Here's how the part is built. I have some questions about the finished solid (model axes, mm). Give positions to 0.01 mm unless a question says otherwise; leave off trailing zeros. Order: outer loops, then holes, each group sorted by start corner. A loop starts at its lowest first (then second) coordinate and runs counter-clockwise, first axis right, second up. Notation, with made-up numbers: M 4.5,56.25 L 40.5,56.25 A22 ccw 40.5,89.25 Z; hole C 61,56 d2. An arc over 180 degrees is marked long. One line per item, written item: value. Start each with the question number.
from build123d import *

# Parameters (mm, degrees)
SKETCH1_R           = 1.5
SKETCH1_R_2         = 3.75
BOSS_EXTRUDE1_DEPTH = 3


with BuildPart() as part:
    # Sketch1 → Boss-Extrude1 (new body)
    # profile 1 of 3: a face of its own
    with BuildSketch(Plane.XY):
        with BuildLine():
            Line((40, 3.75), (0, 3.75))
            ThreePointArc((0, 3.75), (2.651650429, 2.651650429), (3.75, 0))
            ThreePointArc((3.75, 0), (2.651650429, -2.651650429), (0, -3.75))
            Line((0, -3.75), (40, -3.75))
            ThreePointArc((40, -3.75), (36.25, 0), (40, 3.75))
        make_face()
        with Locations((32, 0)):
            Circle(SKETCH1_R, mode=Mode.SUBTRACT)
    # profile 2 of 3: a face of its own
    with BuildSketch(Plane.XY):
        Circle(SKETCH1_R_2)
        Circle(SKETCH1_R, mode=Mode.SUBTRACT)
    # profile 3 of 3: a face of its own
    with BuildSketch(Plane.XY):
        with Locations((40, 0)):
            Circle(SKETCH1_R_2)
        with Locations((40, 0)):
            Circle(SKETCH1_R, mode=Mode.SUBTRACT)
    extrude(amount=BOSS_EXTRUDE1_DEPTH)


solid = part.part
Item 1: I want a section at C-C on x = 32. Write out the boundary of the cut face in (y, z).
Item 2: I want a section at B-B on y = 0. Write out the boundary of the cut face in (x, z), plus the area to 4 significant figures.
Item 3: I want a section at A-A on z = 1.15. Write out the boundary of the cut face in (x, y), plus the area to 3 significant figures.
Item 4: Please list where these lines run through material, in increasing order: probe 1 along Y at (x, z) = (40, 2.15); probe 2 along X at (y, z) = (0.25, 0.4); probe 3 along X at (y, z) = (1.25, 0.6). Write a range as [from, to].
Item 5: I want a section at D-D on y = -2.75. Write out the boundary of the cut face in (x, z), plus the area to 3 significant figures.
Item 6: We'd pull the mould along X, two halves only. Please class faces 1 (the face through (43.75, -0.08, 1.48)), 2 (the face through (20, 3.75, 1)), 3 (the face through (38.5, 0.07, 1.48)): +X half, -X half, draft (parallel to the pull), parting line (faces both ways), or undercut.
Answer below:
1. outline: M -3.75,0 L -1.5,0 L -1.5,3 L -3.75,3 Z; M 1.5,0 L 3.75,0 L 3.75,3 L 1.5,3 Z
2. outline: M -3.75,0 L -1.5,0 L -1.5,3 L -3.75,3 Z; M 1.5,0 L 30.5,0 L 30.5,3 L 1.5,3 Z; M 33.5,0 L 38.5,0 L 38.5,3 L 33.5,3 Z; M 41.5,0 L 43.75,0 L 43.75,3 L 41.5,3 Z
2. area: 115.5 mm²
3. outline: M 0,-3.75 L 40,-3.75 A3.75 ccw 40,3.75 L 0,3.75 A3.75 ccw Z; hole C 0,0 d3; hole C 32,0 d3; hole C 40,0 d3
3. area: 323 mm²
4. probe 1: y = [-3.75, -1.5], [1.5, 3.75]
4. probe 2: x = [-3.74, -1.48], [1.48, 30.52], [33.48, 38.52], [41.48, 43.74]
4. probe 3: x = [-3.54, -0.83], [0.83, 31.17], [32.83, 39.17], [40.83, 43.54]
5. outline: M -2.55,0 L 42.55,0 L 42.55,3 L -2.55,3 Z
5. area: 135 mm²
6. face 1: +X half
6. face 2: draft
6. face 3: undercut
